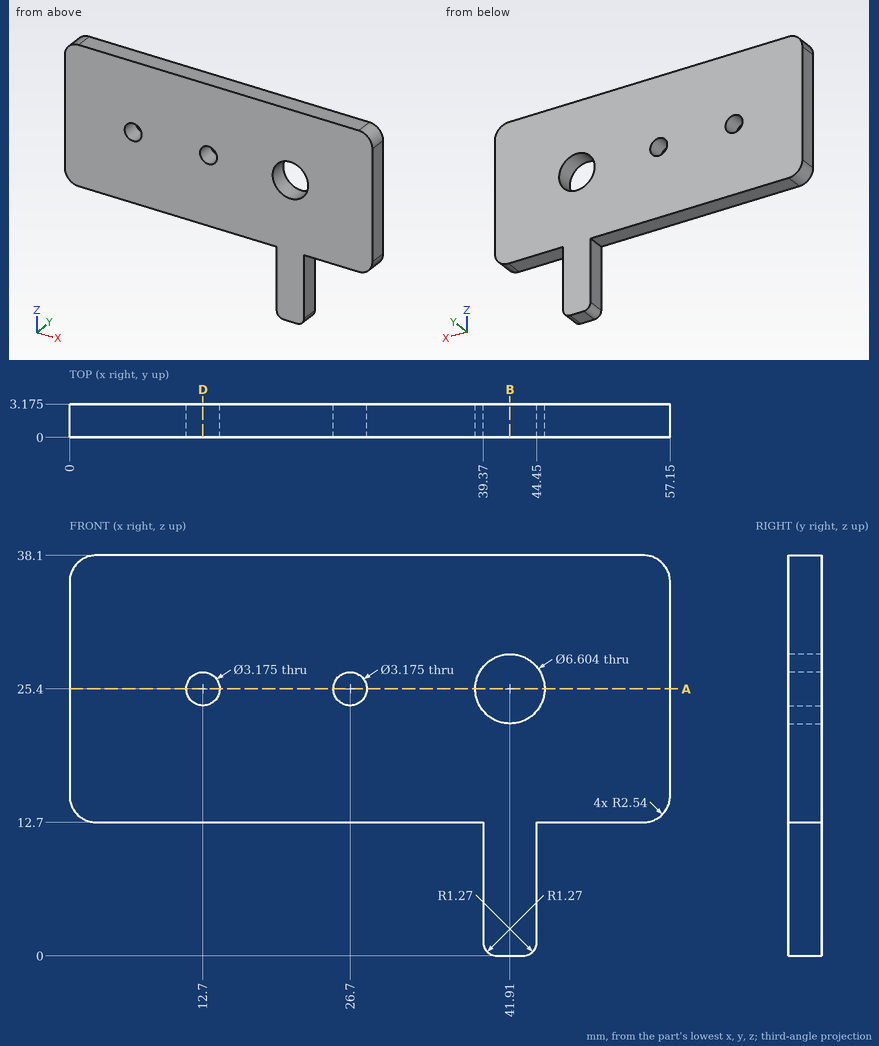
Geometry: see drawing. Coordinates: mm, zero at the bounding-box minimum. Coordinates: 2 decimals unless noted, no trailing zeros. Write each loop counter-clockwise with the first axis right and the second up, starting at its lowest first coordinate (ties: lowest second). Pieces come first, ordered by that corner, then holes. Notation, with made-up numbers: (58.25, -28) - (98.25, -28) arc R27 cw to (98.25, 1) - close; hole circle Ø8 at (6, 13.5). An arc over 180 degrees is marked (long way). Put each result on its own line as item: value. Start each with the question number.
1) Cut plane A-A (z = 25.4). State how many separate pieces and enclosed holes the cut face has, plus the area to 3 significant figures.
2) Cut plane B-B (x = 41.91). Return the cut outline in (y, z) (3 decimals), plus the area to 4 significant figures.
3) Ray query, L1, parallel to X at y = 1.35, z = 25.4; L2, parallel to Z at x = 15, y = 1.35; L3, parallel to Z at x = 13, y = 2. Return the intervals inside material, ascending.
4) Contact query for flat-ended pins moving along their axis: pin 1 (1.9 mm diameter, centred on x = 26.7, z = 25.4, fed in from +Y); pin 2 (1 mm diameter, centred on x = 45, y = 2, fed in from -Z); pin 3 (1 mm diameter, centred on y = 2, z = 4.5, fed in from +X). Output: stop coordinate, or through.
5) Cut plane D-D (x = 12.7). Return the cut outline in (y, z) (1 decimal), plus the area to 3 significant figures.
Resolved:
1. separate pieces: 4
1. enclosed holes: 0
1. area: 140 mm2
2. outline: (0, 0) - (3.175, 0) - (3.175, 22.098) - (0, 22.098) - close; (0, 28.702) - (3.175, 28.702) - (3.175, 38.1) - (0, 38.1) - close
2. area: 100.0 mm2
3. L1: x = 0 to 11.11, 14.29 to 25.11, 28.29 to 38.61, 45.21 to 57.15
3. L2: z = 12.7 to 38.1
3. L3: z = 12.7 to 23.84, 26.96 to 38.1
4. pin 1: passes through
4. pin 2: stops at z = 12.7
4. pin 3: stops at x = 44.45
5. outline: (0, 12.7) - (3.2, 12.7) - (3.2, 23.8) - (0, 23.8) - close; (0, 27) - (3.2, 27) - (3.2, 38.1) - (0, 38.1) - close
5. area: 70.6 mm2
